For this review, take the finished solid that the model builds, in its own axes (mm). A direction names the side the tool comes from. Round coordinates to 2 decimals unless told otherwise and drop trailing zeros. Write each loop counter-clockwise with the first axis right and the second up, starting at its lowest first coordinate (ties: lowest second). Pieces come first, ordered by that corner, then holes. Notation, with made-up numbers: (0.25, 65.25) -> (53.25, 65.25) arc R23 ccw to (53.25, 93.25) -> close; hole circle Ø7 at (20.5, -2.5). An arc over 180 degrees is marked (long way). Write each question's results on one line, items separated by ' | '. Start each with the question number.
Item 1: The part is to be moulded in two halves that separate along Y. For faces 1 (the cylindrical face through (-0.7, 67.21, 7.59)), 2 (the flat face through (-5, 70.626, 8)), 3 (the flat face through (0, 67, 5.25)), say which applies: +Y half, -Y half, draft (parallel to the pull), parting line (faces both ways), or undercut.
Item 2: Clearance check with flat-ended pins moving along their axes: pin 1 (1 mm diameter, centred on y = 45.5, z = 6.5, fed in from -X); pin 2 (3 mm diameter, centred on x = 72, z = 7, fed in from +Y); pin 3 (15.5 mm diameter, centred on x = -5, y = 67, fed in from -Z). State where each tip first meets the part, or that it passes through.
Item 3: Add section B-B (x = 65). State the section outline as (y, z) points, plus the area to 3 significant figures.
Item 4: Tool access review of faces 4 (the flat face through (69, 5, 5)), 5 (the cylindrical face through (-1.431, 58.112, 2.588)), 6 (the flat face through (76.798, 3, 5)): name each direction out of +Z, -Z, +X, -X, +Y, -Y from which nothing blocks a thin tool from reaching the whole face with its end or side.
Item 5: Add section C-C (y = 42). State the section outline as (x, z) points.
Item 6: To check wall thickness, follow line 1 along Y through (x, z) = (-1.5, 9.25); line 2 along X through (y, z) = (47, 0.5); line 3 along Y through (x, z) = (3, 4.5). State the ranges of each line that lie inside material, in increasing order.
Item 7: Add section A-A (z = 2.25). State the section outline as (x, y) points, plus the area to 3 significant figures.
from build123d import *

# Parameters (mm, degrees)
SKETCH_R     = 4.25
PAD_DEPTH    = 10
POCKET_DEPTH = 5.25


with BuildPart() as part:
    # Sketch → Pad (new body)
    with BuildSketch(Plane.XY):
        with BuildLine():
            ThreePointArc((57.5, 0), (36.960288, 44.047555), (-9.98477, 56.626446))
            Line((-9.98477, 56.626446), (-9.98477, 70.626446))
            Line((0, 70.626446), (-9.98477, 70.626446))
            Line((0, 70.626446), (11.447938, 60.933937))
            ThreePointArc((61.798058, 5), (46.080314, 41.480172), (11.447938, 60.933937))
            Line((61.798058, 5), (76.798058, 5))
            Line((76.798058, 5), (76.798058, 0))
            Line((76.798058, 0), (57.5, 0))
        make_face()
        with Locations((-2.98477, 63.626446)):
            Circle(SKETCH_R, mode=Mode.SUBTRACT)
    extrude(amount=PAD_DEPTH)

    # Sketch001 (on Face10 of Pad) → Pocket (cut)
    with BuildSketch(Plane(origin=(0, 0, 0), x_dir=(1, 0, 0), z_dir=(0, 0, -1))):
        with BuildLine():
            ThreePointArc((-10.105268, -56.323298), (-2.630648, -57.953028), (5, -58.5))
            Line((5, -58.5), (11.780711, -62.745227))
            Line((4.894732, -71.323298), (11.780711, -62.745227))
            Line((-10.105268, -71.323298), (4.894732, -71.323298))
            Line((-10.105268, -56.323298), (-10.105268, -71.323298))
        make_face()
    extrude(amount=-POCKET_DEPTH, mode=Mode.SUBTRACT)


solid = part.part
Responses:
1) face 1: undercut | face 2: +Y half | face 3: draft
2) pin 1: stops at x = 34.5 | pin 2: stops at y = 5 | pin 3: stops at z = 5.25
3) outline: (0, 0) -> (5, 0) -> (5, 10) -> (0, 10) -> close | area: 50.0 mm^2
4) face 4: +Z, -Z, +X, +Y | face 5: -Z, -X, +Y | face 6: +Z, -Z, +X, +Y, -Y
5) outline: (39.27, 0) -> (45.61, 0) -> (45.61, 10) -> (39.27, 10) -> close
6) line 1: y = 57.48 to 59.64, 67.61 to 70.63 | line 2: x = 33.12 to 40.44 | line 3: y = 57.42 to 58.46
7) outline: (-7.6, 57) arc R57.5 cw to (57.5, 0) -> (76.8, 0) -> (76.8, 5) -> (61.8, 5) arc R62 ccw to (11.45, 60.93) -> (10.36, 61.86) -> (5, 58.5) arc R53.5 ccw to start | area: 475 mm^2
